from build123d import *

# Parameters (mm, degrees)
F1_DEPTH = 5.08
F3_DEPTH = 5.081
F5_DEPTH = 5.08


with BuildPart() as f1:
    # F0 (on Front) → F1 (new body)
    with BuildSketch(Plane.XZ):
        Polygon((0, 4.306565316), (5.132364687, 0), (219.075, 0), (219.075, 95.25), (5.132364687, 95.25), (0, 90.943434684), align=None)
    extrude(amount=F1_DEPTH)

    # F2 (on face) → F3 (cut, through all)
    with BuildSketch(Plane.XZ.offset(5.08)):
        with BuildLine():
            Line((12.7, 57.15), (12.7, 38.1))
            ThreePointArc((12.7, 38.1), (20.1394877579, 20.1394877579), (38.1, 12.7))
            Line((38.1, 12.7), (180.975, 12.7))
            ThreePointArc((180.975, 12.7), (198.9355122421, 20.1394877579), (206.375, 38.1))
            Line((206.375, 38.1), (206.375, 57.15))
            ThreePointArc((206.375, 57.15), (198.9355122421, 75.1105122421), (180.975, 82.55))
            Line((180.975, 82.55), (38.1, 82.55))
            ThreePointArc((38.1, 82.55), (20.1394877579, 75.1105122421), (12.7, 57.15))
        make_face()
    extrude(amount=-F3_DEPTH, mode=Mode.SUBTRACT)

    # F4 (on face) → F5 (join)
    with BuildSketch(Plane.XZ.offset(5.08)):
        Polygon((212.725, -12.7), (219.075, -12.7), (219.075, 0), (206.375, 0), (206.375, -6.35), align=None)
        Polygon((206.375, 95.25), (219.075, 95.25), (219.075, 107.95), (212.725, 107.95), (206.375, 101.6), align=None)
        Polygon((206.375, 0), (219.075, 0), (219.075, 95.25), (206.375, 95.25), (206.375, 57.15), (206.375, 38.1), align=None)
    extrude(amount=-F5_DEPTH)


solid = f1.part
Could you check a few things on this model? Use its own coordinates, in mm. A direction names the side the tool comes from. Give positions to 0.01 mm unless a question says otherwise; leave off trailing zeros. Write each loop counter-clockwise with the first axis right and the second up, starting at its lowest first coordinate (ties: lowest second). Pieces come first, ordered by that corner, then holes. Notation, with made-up numbers: (-33, 77) -> (8, 77) arc R10 ccw to (8, 88) -> close; hole circle Ø7 at (3, 50). An arc over 180 degrees is marked (long way). Answer as CSV lines item,"result". Start each with the question number.
(1) Please list where these lines run through material, in increasing order: line 1 (Z direction, x = 151.5, y = -0.45); line 2 (X direction, y = -4.55, z = 42.5) (3 decimals).
(2) If we section it at A-A, the plane x = 116: Write out the boundary of the cut face in (y, z).
(3) If we section it at B-B, the plane y = -2.8: Write out the boundary of the cut face in (x, z) (3 decimals).
(4) Which directions (+Z, -Z, +X, -X, +Y, -Y) give clear straight access to the entire face, cutting with the end or side of a thin tool? Please do faces 1 (the face through (20.34, -2.58, 75.31)), 2 (the face through (107, -3, 95.25)), 3 (the face through (216, -3, -12.7)).
(5) If we section it at C-C, the plane z = 73: Write out the boundary of the cut face in (x, y) (3 decimals), and give its area (3 significant figures).
(6) I'm going to push flat-ended pins straight in: pin 1 Ø3 at (x, y) = (74.5, -1) entering from -Z; pin 2 Ø3 at (x, z) = (133, 92) entering from +Y; pin 3 Ø1.5 at (x, y) = (61, -2) entering from +Z. Where does each tip first touch, or does it pass through?
(7) If we mould it in two halves opening along Z, with no side actions, what happens to faces 4 (the face through (198.737, -2.576, 19.943)), 5 (the face through (199.132, -2.576, 74.912)), 6 (the face through (2.53, -2.504, 2.183)), 7 (the face through (206.375, -3, -3))? For each: +Z half, -Z half, draft (parallel to the pull), parting line (faces both ways), or undercut.
Answer list:
1,line 1,"0 to 12.7, 82.55 to 95.25"
1,line 2,"0 to 12.7, 206.375 to 219.075"
2,outline,"(-5.08, 0) -> (0, 0) -> (0, 12.7) -> (-5.08, 12.7) -> close; (-5.08, 82.55) -> (0, 82.55) -> (0, 95.25) -> (-5.08, 95.25) -> close"
3,outline,"(0, 4.307) -> (5.132, 0) -> (206.375, 0) -> (206.375, -6.35) -> (212.725, -12.7) -> (219.075, -12.7) -> (219.075, 107.95) -> (212.725, 107.95) -> (206.375, 101.6) -> (206.375, 95.25) -> (5.132, 95.25) -> (0, 90.943) -> close; hole (12.7, 38.1) arc R25.4 ccw to (38.1, 12.7) -> (180.975, 12.7) arc R25.4 ccw to (206.375, 38.1) -> (206.375, 57.15) arc R25.4 ccw to (180.975, 82.55) -> (38.1, 82.55) arc R25.4 ccw to (12.7, 57.15) -> close"
4,face 1,"+Y, -Y"
4,face 2,"+Z, -X, +Y, -Y"
4,face 3,"-Z, +X, -X, +Y, -Y"
5,outline,"(0, -5.08) -> (18.252, -5.08) -> (18.252, 0) -> (0, 0) -> close; (200.823, -5.08) -> (219.075, -5.08) -> (219.075, 0) -> (200.823, 0) -> close"
5,area,"185 mm^2"
6,pin 1,"z = 0"
6,pin 2,"y = 0"
6,pin 3,"z = 95.25"
7,face 4,"undercut"
7,face 5,"undercut"
7,face 6,"-Z half"
7,face 7,"draft"
